from build123d import *

# Parameters (mm, degrees)
SKETCH_1_W          = 30
SKETCH_1_H          = 6
EXTRUDE_1_DEPTH     = 2
SKETCH_2_R          = 0.8
CUT_EXTRUDE_1_DEPTH = 2
SKETCH_3_W          = 1.6
SKETCH_3_H          = 0.2
EXTRUDE_2_DEPTH     = 10
SKETCH_4_W          = 21.8
SKETCH_4_H          = 0.2
EXTRUDE_3_DEPTH     = 1.6
SKETCH_5_W          = 5
SKETCH_5_H          = 0.2
EXTRUDE_4_DEPTH     = 10
SKETCH_6_W          = 5.4
SKETCH_6_H          = 7.2
EXTRUDE_5_DEPTH     = 5.4
FILLET_1_R          = 2
SKETCH_7_R          = 0.8
CUT_EXTRUDE_2_DEPTH = 32.429922049
SKETCH_8_W          = 6
SKETCH_8_H          = 2
CUT_EXTRUDE_3_DEPTH = 33.86335345
SKETCH_9_W          = 21.8
SKETCH_9_H          = 1.6
EXTRUDE_7_DEPTH     = 0.2
EXTRUDE_9_DEPTH     = 1.6
EXTRUDE_10_REACH    = 49.608
EXTRUDE_11_DEPTH    = 1.6
CUT_EXTRUDE_4_DEPTH = 1.6
FILLET_2_R          = 9
FILLET_3_R          = 9.5
FILLET_4_R          = 1
CHAMFER_1_SIZE      = 12.342759107
CHAMFER_1_SIZE_2    = 5


with BuildPart() as part:
    # 草图1 → 凸台-拉伸1 (new body)
    with BuildSketch(Plane(origin=(0, 0, 0), x_dir=(1, 0, 0), z_dir=(0, 1, 0))):
        with Locations((15, -3)):
            Rectangle(SKETCH_1_W, SKETCH_1_H)
    extrude(amount=EXTRUDE_1_DEPTH)

    # 草图2 → 切除-拉伸1 (cut)
    with BuildSketch(Plane(origin=(0, 2, 0), x_dir=(1, 0, 0), z_dir=(0, 1, 0))):
        with Locations(Location((27.25, -3, 0), (0, 0, 270))):
            Circle(SKETCH_2_R)
    extrude(amount=-CUT_EXTRUDE_1_DEPTH, mode=Mode.SUBTRACT)

    # 草图3 → 凸台-拉伸2 (add)
    with BuildSketch(Plane(origin=(0, 2, 0), x_dir=(1, 0, 0), z_dir=(0, 1, 0))):
        with Locations((0.8, -5.9)):
            Rectangle(SKETCH_3_W, SKETCH_3_H)
        with Locations((24.2, -5.9)):
            Rectangle(SKETCH_3_W, SKETCH_3_H)
    extrude(amount=EXTRUDE_2_DEPTH)

    # 草图4 → 凸台-拉伸3 (add)
    with BuildSketch(Plane(origin=(0, 12, 0), x_dir=(1, 0, 0), z_dir=(0, 1, 0))):
        with Locations((12.5, -5.9)):
            Rectangle(SKETCH_4_W, SKETCH_4_H)
    extrude(amount=-EXTRUDE_3_DEPTH)

    # 草图5 → 凸台-拉伸4 (add)
    with BuildSketch(Plane(origin=(0, 2, 0), x_dir=(1, 0, 0), z_dir=(0, 1, 0))):
        with Locations((27.5, -5.9)):
            Rectangle(SKETCH_5_W, SKETCH_5_H)
    extrude(amount=EXTRUDE_4_DEPTH)

    # 草图6 → 凸台-拉伸5 (add)
    with BuildSketch(Plane(origin=(0, 0, 5.8), x_dir=(-1, 0, 0), z_dir=(0, 0, -1))):
        with Locations((-27.3, 8.4)):
            Rectangle(SKETCH_6_W, SKETCH_6_H)
    extrude(amount=EXTRUDE_5_DEPTH)

    # 圆角1
    fillet_1_edges = [part.edges().sort_by_distance(p)[0] for p in [
        (24.6, 8.4, 0.4),
    ]]
    fillet(fillet_1_edges, radius=FILLET_1_R)

    # 草图7 → 切除-拉伸2 (cut, through all)
    with BuildSketch(Plane(origin=(0, 4.8, 0), x_dir=(-1, 0, 0), z_dir=(0, -1, 0))):
        with Locations(Location((-27.25, -3, 0), (0, 0, 270))):
            Circle(SKETCH_7_R)
    extrude(amount=-CUT_EXTRUDE_2_DEPTH, mode=Mode.SUBTRACT)

    # 草图8 → 切除-拉伸3 (cut, through all)
    with BuildSketch(Plane.ZY):
        with Locations((3, 1)):
            Rectangle(SKETCH_8_W, SKETCH_8_H)
    extrude(amount=-CUT_EXTRUDE_3_DEPTH, mode=Mode.SUBTRACT)

    # 草图9 → 凸台-拉伸7 (add)
    with BuildSketch(Plane.XY.offset(6)):
        with Locations((12.5, 2.8)):
            Rectangle(SKETCH_9_W, SKETCH_9_H)
    extrude(amount=-EXTRUDE_7_DEPTH)

    # 草图11 → 凸台-拉伸9 (add)
    with BuildSketch(Plane(origin=(0, 2, 0), x_dir=(-1, 0, 0), z_dir=(0, -1, 0))):
        Polygon((0, -6), (-10, -36), (-20, -36), (-25, -6), align=None)
    extrude(amount=-EXTRUDE_9_DEPTH)

    # 凸台-拉伸10: up to this face of the body (flat: up to its plane)
    extrude_10_end = Plane(part.part.faces().sort_by_distance((25.077544524, 12, 3.686395467))[0])
    # 草图12 → 凸台-拉伸10 (add, up to the picked face)
    with BuildSketch(Plane(origin=(0, 3.6, 0), x_dir=(1, 0, 0), z_dir=(0, 1, 0)), mode=Mode.PRIVATE) as extrude_10_sk1:
        Polygon((2.219881419, -7.6), (11.153214752, -34.4), (18.644596659, -34.4), (23.111263325, -7.6), (23.4, -6), (25, -6), (20, -36), (10, -36), (0, -6), (1.6, -6), align=None)
    extrude_10_tool1 = split(extrude(extrude_10_sk1.sketch, amount=EXTRUDE_10_REACH, mode=Mode.PRIVATE), bisect_by=extrude_10_end, keep=Keep.BOTH, mode=Mode.PRIVATE)
    add(extrude_10_tool1.solids().sort_by(Axis((6.316075, 3.6, 21.123491), (0, 1, 0)))[0])

    # 草图13 → 凸台-拉伸11 (add)
    with BuildSketch(Plane(origin=(0, 12, 0), x_dir=(1, 0, 0), z_dir=(0, 1, 0))):
        Polygon((1.6, -5.8), (1.6, -6), (2.219881419, -7.6), (11.153214752, -34.4), (18.644596659, -34.4), (23.111263325, -7.6), (23.4, -6), (23.4, -5.8), align=None)
    extrude(amount=-EXTRUDE_11_DEPTH)

    # 草图15 → 切除-拉伸4 (cut)
    with BuildSketch(Plane.XZ.offset(-2)):
        Polygon((11.153214752, 34.4), (18.644596659, 34.4), (19.311263325, 30.4), (9.819881419, 30.4), align=None)
    extrude(amount=-CUT_EXTRUDE_4_DEPTH, mode=Mode.SUBTRACT)

    # 圆角2
    # the kernel refuses this fillet: 9 mm, written as the material it adds along each edge
    with BuildSketch(Plane(origin=(-11.296729569, 10.4, 34.4), x_dir=(0, -1, 0), z_dir=(1, 0, 0))) as fillet_2_piece_1_section:
        with BuildLine():
            CenterArc((9, 8.979977728), FILLET_2_R, 180, 86.177446271)
            Line((0, 8.979977728), (-0.18, 8.979977728))
            Line((-0.18, 8.979977728), (-0.18, 0))
            Line((-0.18, 0), (0, -0.18))
            ThreePointArc((0, -0.18), (4.2, -0.18), (8.388, -0.179599555))
            Line((8.388, -0.179599555), (8.4, 0))
        make_face()
    fillet_2_piece_1 = extrude(amount=52.391270548, mode=Mode.PRIVATE)
    fillet_2_piece_1 = split(fillet_2_piece_1, bisect_by=Plane(origin=(10.82791011, 8.54108789, 33.424086075), z_dir=(0.9486832980505115, 0, -0.3162277660168449)), keep=Keep.TOP, mode=Mode.PRIVATE)
    fillet_2_piece_1 = split(fillet_2_piece_1, bisect_by=Plane(origin=(18.906334999, 8.54108789, 32.829569958), z_dir=(-0.9863939238321403, 0, -0.16439898730537805)), keep=Keep.TOP, mode=Mode.PRIVATE)
    add(fillet_2_piece_1)

    # 圆角3
    fillet_3_edges = [part.edges().sort_by_distance(p)[0] for p in [
        (15, 12, 36),
    ]]
    fillet(fillet_3_edges, radius=FILLET_3_R)

    # 圆角4
    fillet_4_edges = [part.edges().sort_by_distance(p)[0] for p in [
        (14.565572372, 3.6, 30.4),
    ]]
    fillet(fillet_4_edges, radius=FILLET_4_R)

    # 倒角1
    # the kernel refuses this chamfer: 12.342759107, 5 mm, written as the material it adds along each edge
    with BuildSketch(Plane(origin=(25, 12, 6), x_dir=(0.9999085325872852, 0, -0.013525030837001994), z_dir=(0, -1, 0))) as chamfer_1_piece_1_section:
        Polygon((CHAMFER_1_SIZE * 0.99990853261, CHAMFER_1_SIZE * 0.0135250308373), (-CHAMFER_1_SIZE_2 * 0.177724958393, CHAMFER_1_SIZE_2 * 0.984080199559), (0, 0), align=None)
    chamfer_1_piece_1 = extrude(amount=10, mode=Mode.PRIVATE)
    chamfer_1_piece_1 = split(chamfer_1_piece_1, bisect_by=Plane(origin=(30, 7, 7.970980812), z_dir=(-1, 0, 0)), keep=Keep.TOP, mode=Mode.PRIVATE)
    add(chamfer_1_piece_1)


solid = part.part
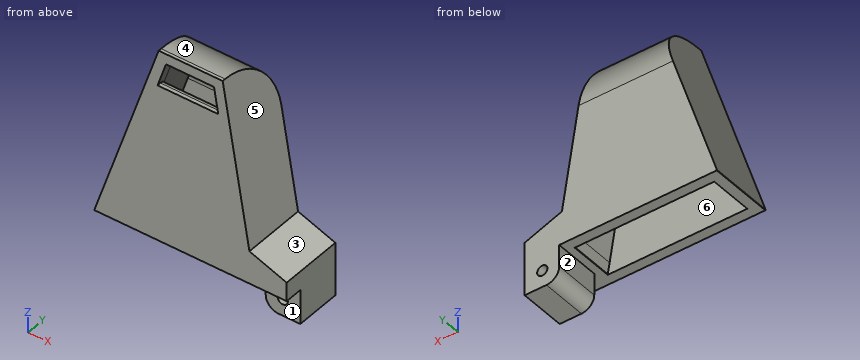
Geometry: final body of the model. Coordinates: model frame, mm. Face numbers are marked on the shaded views. A direction names the side the tool comes from. Round coordinates to 2 decimals unless told otherwise and drop trailing zeros. Loops run counter-clockwise (first coordinate to the right, second up) from the corner with the lowest first, then second, coordinate; pieces in that order, holes last. Notation, with made-up numbers: (8, 70.5) - (39, 70.5) arc R29 cw to (39, 90.5) - close; hole circle Ø1 at (72, 54). An arc over 180 degrees is marked (long way). Write each question's results on one line, items separated by ' | '. Start each with the question number.
1) Mould query, pull axis X, two halves, no side actions, for the marked faces 4, 5 and 6. Classes: released by +X, released by -X, zero draft, split by the parting line, or undercut.
2) Cut plane B-B on z = 3. Return loops of the section in (x, y), then the cut area to 3 significant figures.
3) Line query: probe 1 along Y at (x, z) = (14, 13.5); probe 2 along X at (y, z) = (7, 3); probe 3 along X at (y, z) = (5, 14). Output: solid intervals per line, ascending. Write a range as [from, to].
4) Cut plane C-C on y = 6. Return loops of the section in (x, z).
5) Access query for the marked faces 1, 2 and 3. Directions: +Z, -Z, +X, -X, +Y, -Y. A direction counts if a zero-diameter tool reaches every point of the face in a straight line with its end or side. Return the directions, or none.
6) Cut plane D-D on z = 15. Return loops of the section in (x, y), then the cut area to 3 significant figures.
7) First-contact query: P1, Ø10, axis at x = 24.5, z = 30, coming from the -Y side; P2, Ø6, axis at x = 26.5, z = 2.5, coming from the -Y side; P3, Ø4, axis at x = 14, y = 4.5, coming from the -Z side; P4, Ø3.5, axis at y = 9.5, z = 4, coming from the -X side. Flat tips, straight axial feed; report the tip coordinate or a pass-through.
8) Cut plane A-A on x = 17.5. Return loops of the section in (y, z).
Verdict:
1) face 4: zero draft | face 5: released by +X | face 6: undercut
2) outline: (24.6, 4.8) - (26.45, 4.8) - (26.45, 12) - (24.6, 12) - close; (28.05, 4.8) - (30, 4.8) - (30, 12) - (28.05, 12) - close | area: 27.4 mm2
3) probe 1: y = [2, 3.6], [10.4, 12] | probe 2: x = [24.6, 26.45], [28.05, 30] | probe 3: x = [2.67, 4.35], [22.04, 23.67]
4) outline: (0, 5.8) - (1.6, 5.8) - (1.6, 6) - (2.22, 7.6) - (10.74, 33.16) - (18.85, 33.16) - (23.11, 7.6) - (23.4, 6) - (23.4, 5.8) - (24.6, 5.8) - (24.6, 2.4) arc R2 ccw to (26.6, 0.4) - (30, 0.4) - (30, 8.75) - (24.18, 10.93) - (20.11, 35.33) - (9.78, 35.33) - (0, 6) - close; hole circle Ø1.6 at (27.25, 3)
5) face 1: -Z, +X, -X, -Y | face 2: -Z, -X, +Y, -Y | face 3: +Z, +X, +Y, -Y
6) outline: (3, 2) - (23.5, 2) - (23.5, 12) - (3, 12) - close; hole (4.69, 3.6) - (21.88, 3.6) - (21.88, 10.4) - (4.69, 10.4) - close | area: 88.1 mm2
7) P1: stops at y = 2 | P2: stops at y = 4.8 | P3: stops at z = 5.8 | P4: stops at x = 24.6
8) outline: (2, 5.8) - (3.6, 5.8) - (3.6, 29.4) arc R1 ccw to (2.6, 30.4) - (2, 30.4) - close; (2, 34.4) arc R9 cw to (10.4, 25.42) - (10.4, 5.8) - (12, 5.8) - (12, 26.5) arc R9.5 ccw to (2.5, 36) - (2, 36) - close
